The model under review builds one solid part; all positions refer to its coordinate system, in mm. A direction names the side the tool comes from. Round coordinates to 2 decimals unless told otherwise and drop trailing zeros. Loops run counter-clockwise (first coordinate to the right, second up) from the corner with the lowest first, then second, coordinate; pieces in that order, holes last. Notation, with made-up numbers: (29, 57) - (49, 57) arc R22 cw to (49, 96) - close; hole circle Ø6 at (-10.75, 58). An arc over 180 degrees is marked (long way). Answer as CSV lines item,"result".
from build123d import *

# Parameters (mm, degrees)
SALIENTE_EXTRUIR2_DEPTH    = 15
CORTAR_EXTRUIR5_START      = -126
CORTAR_EXTRUIR5_DEPTH      = 126
CORTAR_EXTRUIR6_DEPTH      = 13
SALIENTE_EXTRUIR3_DEPTH    = 1
SALIENTE_EXTRUIR4_DEPTH    = 1
CORTAR_EXTRUIR7_DEPTH      = 122
SALIENTE_EXTRUIR5_DEPTH    = 2
SALIENTE_EXTRUIR6_DEPTH    = 16
CORTAR_EXTRUIR8_DEPTH      = 180
CORTAR_EXTRUIR8_DEPTH_BACK = 180
CROQUIS12_R                = 2


# Read off the part's stored shape, not the designer's step: Cortar-Extruir5
with BuildPart() as part:
    # Croquis1 → Saliente-Extruir2 (new body)
    with BuildSketch(Plane(origin=(0, 0, 0), x_dir=(1, 0, 0), z_dir=(0, 1, 0))):
        with BuildLine():
            Line((0, 0), (2, 0))
            Line((2, 0), (2, -11))
            Line((2, -11), (128, -11))
            Line((128, -11), (128, 0))
            Line((128, 0), (130, 0))
            Line((130, 0), (130, 187))
            ThreePointArc((130, 187), (128.828427125, 189.828427125), (126, 191))
            Line((126, 191), (4, 191))
            ThreePointArc((4, 191), (1.171572875, 189.828427125), (0, 187))
            Line((0, 187), (0, 0))
        make_face()
    extrude(amount=SALIENTE_EXTRUIR2_DEPTH)

    # Cortar-Extruir5 outline → Cortar-Extruir5 (cut)
    with BuildSketch(Plane(origin=(128, 0, 0), x_dir=(0, 0, -1), z_dir=(1, 0, 0)).offset(CORTAR_EXTRUIR5_START)):
        with BuildLine():
            Line((-11, 0), (-3.5, 0))
            ThreePointArc((-3.5, 0), (-8.803300859, 2.196699141), (-11, 7.5))
            Line((-11, 7.5), (-11, 0))
        make_face()
        with BuildLine():
            Line((-11, 15), (-11, 7.5))
            ThreePointArc((-11, 7.5), (-8.803300859, 12.803300859), (-3.5, 15))
            Line((-3.5, 15), (-11, 15))
        make_face()
    extrude(amount=CORTAR_EXTRUIR5_DEPTH, mode=Mode.SUBTRACT)

    # Croquis3 → Cortar-Extruir6 (cut)
    with BuildSketch(Plane(origin=(0, 15, 0), x_dir=(1, 0, 0), z_dir=(0, 1, 0))):
        with BuildLine():
            Line((2, 80.037921952), (2, 185))
            ThreePointArc((2, 185), (3.171572875, 187.828427125), (6, 189))
            Line((6, 189), (124, 189))
            ThreePointArc((124, 189), (126.828427125, 187.828427125), (128, 185))
            Line((128, 185), (128, 95.850744251))
            Line((128, 95.850744251), (128, 2))
            Line((128, 2), (126, 2))
            Line((126, 2), (126, -1.75))
            Line((126, -1.75), (57.409845297, -1.5))
            Line((57.409845297, -1.5), (4, -1.75))
            Line((4, -1.75), (4, 2))
            Line((4, 2), (2, 2))
            Line((2, 2), (2, 80.037921952))
        make_face()
    extrude(amount=-CORTAR_EXTRUIR6_DEPTH, mode=Mode.SUBTRACT)

    # Croquis6 → Saliente-Extruir3 (add)
    with BuildSketch(Plane.ZY.offset(-128)):
        Polygon((-183, 15), (-8, 15), (-11, 18), (-180, 18), align=None)
    extrude(amount=-SALIENTE_EXTRUIR3_DEPTH)

    # Croquis7 → Saliente-Extruir4 (add)
    with BuildSketch(Plane(origin=(2, 0, 0), x_dir=(0, 0, -1), z_dir=(1, 0, 0))):
        Polygon((183, 15), (180, 18), (11, 18), (8, 15), align=None)
    extrude(amount=-SALIENTE_EXTRUIR4_DEPTH)

    # Croquis8 → Cortar-Extruir7 (cut)
    with BuildSketch(Plane(origin=(4, 0, 0), x_dir=(0, 0, -1), z_dir=(1, 0, 0))):
        with BuildLine():
            Line((-3.5, 13), (5.32233659, 13))
            Line((5.32233659, 13), (5.32233659, 2))
            Line((5.32233659, 2), (-3.5, 2))
            ThreePointArc((-3.5, 2), (-9, 7.5), (-3.5, 13))
        make_face()
    extrude(amount=CORTAR_EXTRUIR7_DEPTH, mode=Mode.SUBTRACT)

    # Croquis10 → Saliente-Extruir5 (add)
    with BuildSketch(Plane.XY.offset(-189)):
        Polygon((65, 2), (73, 2), (73, 19), (72.859656946, 19), (57, 19), (57, 2), align=None)
    extrude(amount=SALIENTE_EXTRUIR5_DEPTH)

    # Croquis11 → Saliente-Extruir6 (add)
    with BuildSketch(Plane(origin=(73, 0, 0), x_dir=(0, 0, -1), z_dir=(1, 0, 0))):
        with BuildLine():
            Line((189, 19.00862759), (189, 16.20862759))
            ThreePointArc((189, 16.20862759), (190.4, 17.60862759), (189, 19.00862759))
        make_face()
    extrude(amount=-SALIENTE_EXTRUIR6_DEPTH)

    # Croquis12 → Cortar-Extruir8 (cut, two sides: drawn at the far end of the back side and taken through both)
    with BuildSketch(Plane(origin=(4, 0, 0), x_dir=(0, 0, -1), z_dir=(1, 0, 0)).offset(-CORTAR_EXTRUIR8_DEPTH_BACK)):
        with Locations(Location((-3.5, 7.5, 0), (0, 0, 180))):
            Circle(CROQUIS12_R)
    extrude(amount=CORTAR_EXTRUIR8_DEPTH + CORTAR_EXTRUIR8_DEPTH_BACK, mode=Mode.SUBTRACT)


solid = part.part
1. Take a section at C-C (x = 90). State the section outline as (y, z) points.
Numbers:
outline,"(0, -191) - (15, -191) - (15, -189) - (2, -189) - (2, 3.5) arc R5.5 cw to (13, 3.5) - (13, 1.62) - (15, 1.62) - (15, 3.5) arc R7.5 ccw to (0, 3.5) - close"
2. Take a section at A-A (x = 40.5). State the section outline as (y, z) points, plus the area to 3 significant figures.
Numbers:
outline,"(0, -191) - (15, -191) - (15, -189) - (2, -189) - (2, 3.5) arc R5.5 cw to (13, 3.5) - (13, 1.58) - (15, 1.58) - (15, 3.5) arc R7.5 ccw to (0, 3.5) - close"
area,"460 mm²"
3. Take a section at B-B (z = -23.5). State the section outline as (x, y) points.
Numbers:
outline,"(0, 0) - (130, 0) - (130, 15) - (129, 15) - (129, 18) - (128, 18) - (128, 2) - (2, 2) - (2, 18) - (1, 18) - (1, 15) - (0, 15) - close"
4. Tool access review of faces 1 (the face through (98, 9, -189)), 2 (the face through (126, 9, 1)), 3 (the face through (2, 9.1, 5.4)): name each direction out of +Z, -Z, +X, -X, +Y, -Y from which nothing blocks a thin tool from reaching the whole face with its end or side.
Numbers:
face 1,"+Y"
face 2,"none"
face 3,"+Z, -X, +Y, -Y"
5. Clearance check with flat-ended pins moving along their axes: pin 1 (1 mm diameter, centred on y = 8.5, z = -189.5, fed in from +X); pin 2 (0.5 mm diameter, centred on x = 1.5, z = -100, fed in from +Y); pin 3 (1 mm diameter, centred on x = 129.5, y = 6.5, fed in from +Z). State where each tip first meets the part, or that it passes through.
Numbers:
pin 1,"stops at x = 129.46"
pin 2,"stops at y = 18"
pin 3,"stops at z = 0"
6. Wall thickness on probe 1 along X at (y, z) = (11.25, -81.5); probe 2 along Y at (x, z) = (66.5, -75); probe 3 along Z at (x, y) = (69.5, 9.5): over which ranges is each line inside the solid? List them lowest first.
Numbers:
probe 1,"x = 0 to 2, 128 to 130"
probe 2,"y = 0 to 2"
probe 3,"z = -191 to -187, 8.62 to 10.73"
7. Draft analysis for pull direction Z (two halves, no side actions). For faces 4 (the face through (64, 0, -95)), 5 (the face through (31, 9, -189)), 6 (the face through (1.203, 7.395, -189.859)), state which applies: +Z half, -Z half, draft (parallel to the pull), parting line (faces both ways), or undercut.
Numbers:
face 4,"draft"
face 5,"undercut"
face 6,"-Z half"
